```python
from build123d import *

# Parameters (mm, degrees)
SKETCH4_R               = 2.05
SKETCH4_W               = 5
SKETCH4_H               = 20
BOSS_LARGEUR_DEPTH      = 10
SKETCH4_4_W             = 5
SKETCH4_4_H             = 20
BOSS_EXTRUDE4_DEPTH     = 8
CUT_VIS_REACH           = 36.848
SKETCH5_R               = 2.1
SKETCH5_R_2             = 4
SKETCH5_4_R             = 4
SKETCH5_4_R_2           = 2.1
BOSS_VIS_DEPTH          = 8
SKETCH4_6_R             = 2.05
CUT_EXTRUDE7_DEPTH      = 27
CUT_EXTRUDE7_DEPTH_BACK = 5


with BuildPart() as part:
    # Sketch4 → Boss-Largeur (new body)
    with BuildSketch(Plane.XY):
        with BuildLine():
            Line((40, 10), (-10, 10))
            ThreePointArc((-10, 10), (-13.535533906, 8.535533906), (-15, 5))
            Line((-15, 5), (-15, -5))
            ThreePointArc((-15, -5), (-13.535533906, -8.535533906), (-10, -10))
            Line((-10, -10), (40, -10))
            Line((40, -10), (40, 10))
        make_face()
        Circle(SKETCH4_R, mode=Mode.SUBTRACT)
        with Locations((42.5, 0)):
            Rectangle(SKETCH4_W, SKETCH4_H)
        Polygon((75, -1.961524227), (45, 10), (45, -10), align=None)
        Circle(SKETCH4_R)
    extrude(amount=-BOSS_LARGEUR_DEPTH)

    # Sketch4<4> → Boss-Extrude4 (add)
    with BuildSketch(Plane.XY):
        with Locations((42.5, 0)):
            Rectangle(SKETCH4_4_W, SKETCH4_4_H)
        Polygon((45, -10), (75, -1.961524227), (45, 10), align=None)
    extrude(amount=BOSS_EXTRUDE4_DEPTH)

    # Sketch5 → Cut-Vis (cut, up to next)
    with BuildSketch(Plane(origin=(5.514428415, -20.580127019, 0), x_dir=(0.965925826, 0.258819045, 0), z_dir=(0.258819045, -0.965925826, 0)), mode=Mode.PRIVATE) as cut_vis_sk1:
        with Locations((56.936757144, -2)):
            Circle(SKETCH5_R)
    cut_vis_tool1 = extrude(cut_vis_sk1.sketch, amount=-CUT_VIS_REACH, mode=Mode.PRIVATE) & part.part
    add(cut_vis_tool1.solids().sort_by_distance((60.511113, -5.84381, -2))[0], mode=Mode.SUBTRACT)
    # Sketch5 → Cut-Vis (cut, up to next)
    with BuildSketch(Plane(origin=(5.514428415, -20.580127019, 0), x_dir=(0.965925826, 0.258819045, 0), z_dir=(0.258819045, -0.965925826, 0)), mode=Mode.PRIVATE) as cut_vis_sk2:
        with Locations((56.936757144, -2)):
            Circle(SKETCH5_R_2)
        with Locations((56.936757144, -2)):
            Circle(SKETCH5_R, mode=Mode.SUBTRACT)
    cut_vis_tool2 = extrude(cut_vis_sk2.sketch, amount=-CUT_VIS_REACH, mode=Mode.PRIVATE) & part.part
    add(cut_vis_tool2.solids().sort_by_distance((56.756691, -6.849804, -2))[0], mode=Mode.SUBTRACT)

    # Sketch5<4> → Boss-Vis (add)
    with BuildSketch(Plane(origin=(5.514428415, -20.580127019, 0), x_dir=(0.965925826, 0.258819045, 0), z_dir=(0.258819045, -0.965925826, 0))):
        with Locations((56.936757144, -2)):
            Circle(SKETCH5_4_R)
        with Locations((56.936757144, -2)):
            Circle(SKETCH5_4_R_2, mode=Mode.SUBTRACT)
    extrude(amount=-BOSS_VIS_DEPTH)

    # Mirror4: part across plane


with BuildPart() as part_1:
    add(part.part)
    add(part.part.mirror(Plane.XY.offset(8)))

    # Sketch4<6> → Cut-Extrude7 (cut, two sides)
    with BuildSketch(Plane.XY) as cut_extrude7_sk:
        Circle(SKETCH4_6_R)
    extrude(amount=CUT_EXTRUDE7_DEPTH, mode=Mode.SUBTRACT)
    extrude(cut_extrude7_sk.sketch, amount=-CUT_EXTRUDE7_DEPTH_BACK, mode=Mode.SUBTRACT)


solid = part_1.part
```
Geometry: final body of the model. Coordinates: model frame, mm. A direction names the side the tool comes from. Round coordinates to 2 decimals unless told otherwise and drop trailing zeros. Order: outer loops, then holes, each group sorted by start corner. A loop starts at its lowest first (then second) coordinate and runs counter-clockwise, first axis right, second up. Notation, with made-up numbers: (4.25, -21.5) -> (57.25, -21.5) arc R23 ccw to (57.25, 1.5) -> close; hole circle Ø2 at (-22.5, -16). An arc over 180 degrees is marked (long way). Use one line per item in the form item = value.
(1) Section C-C on z = 6. Return loops of the section in (x, y), and give its area (3 significant figures).
Results list:
outline = (40, -10) -> (45, -10) -> (75, -1.96) -> (45, 10) -> (40, 10) -> close
area = 400 mm^2
(2) Section B-B on z = -3. Return loops of the section in (x, y).
Results list:
outline = (-15, -5) arc R5 ccw to (-10, -10) -> (45, -10) -> (58.73, -6.32) -> (56.66, 1.41) -> (54.7, 0.88) -> (53.12, 6.76) -> (45, 10) -> (-10, 10) arc R5 ccw to (-15, 5) -> close; (60.22, 2.36) -> (62.29, -5.37) -> (75, -1.96) -> (62.1, 3.18) -> (62.18, 2.89) -> close; hole circle Ø4.1 at (0, 0)
(3) Section D-D on y = 8.5. Return loops of the section in (x, z), and give its area (3 significant figures).
Results list:
outline = (-13.57, -10) -> (48.76, -10) -> (48.76, 26) -> (-13.57, 26) -> (-13.57, 16) -> (40, 16) -> (40, 0) -> (-13.57, 0) -> close
area = 1,390 mm^2
(4) Ray query, probe 1 along Z at (x, y) = (9, -5); probe 2 along Y at (x, z) = (0, -3); probe 3 along Z at (x, y) = (0.5, -0.5). Return the intervals inside material, ascending. Write a range as [from, to].
Results list:
probe_1 = [-10, 0], [16, 26]
probe_2 = [-10, -2.05], [2.05, 10]
probe_3 = [-10, -5]
(5) Draft query along X for faces 4 (the face through (12, 0, 16)), 5 (the face through (-13, 9, -5)), 6 (the face through (54, 3, 18)). Return one class per face: pulls with the +X half, pulls with the -X half, needs draft (parallel to the pull), parting line crosses it, or undercut.
Results list:
face_4 = needs draft
face_5 = pulls with the -X half
face_6 = undercut
(6) First-contact query: pin 1 Ø2 at (x, y) = (0, 0) entering from +Z; pin 2 Ø3 at (x, z) = (53, 21) entering from -Y; pin 3 Ø2 at (x, z) = (54.5, 21) entering from -Y. Flat tips, straight axial feed; report the tip coordinate or a pass-through.
Results list:
pin_1 = -5
pin_2 = -8.26
pin_3 = -7.72
(7) Access query for faces 1 (the face through (19, 0, -10)), 2 (the face through (-0.267, 2.033, -2.465)), 3 (the face through (12, 0, 0)). Directions: +Z, -Z, +X, -X, +Y, -Y. A direction counts if a zero-diameter tool reaches every point of the face in a straight line with its end or side. Return the directions, or none.
Results list:
face_1 = -Z, +X, -X, +Y, -Y
face_2 = +Z
face_3 = -X, +Y, -Y
(8) Section A-A on x = 0. Return loops of the section in (y, z).
Results list:
outline = (-10, -10) -> (10, -10) -> (10, 0) -> (2.05, 0) -> (2.05, -5) -> (-2.05, -5) -> (-2.05, 0) -> (-10, 0) -> close; (-10, 16) -> (-2.05, 16) -> (-2.05, 26) -> (-10, 26) -> close; (2.05, 16) -> (10, 16) -> (10, 26) -> (2.05, 26) -> close
